Here's how the part is built. I have some questions about the finished solid (model axes, mm). Face numbers are marked on the shaded views. A direction names the side the tool comes from. Round coordinates to 2 decimals unless told otherwise and drop trailing zeros. Order: outer loops, then holes, each group sorted by start corner. A loop starts at its lowest first (then second) coordinate and runs counter-clockwise, first axis right, second up. Notation, with made-up numbers: M 57.25,-16 L 116.25,-16 A18 cw 116.25,-2 Z; hole C 88.5,49.25 d2. An arc over 180 degrees is marked long. Write each question's results on one line, items separated by ' | '. Start each with the question number.
```python
from build123d import *

# Parameters (mm, degrees)
EXTRUDE_THIN1_DEPTH            = 152.5
CONVERT_SOLID1_START           = -152.5
CONVERT_SOLID1_DEPTH           = 305
CONVERT_SOLID1_2_DEPTH         = 305
FILLET1_R                      = 2
F_6_5_6_5_DIAMETER_HOLE1_D     = 6.5
F_6_5_6_5_DIAMETER_HOLE2_D     = 6.5
F_6_5_6_5_DIAMETER_HOLE2_DEPTH = 497


# Read off the part's stored shape, not the designer's step: Convert-Solid1
with BuildPart() as part:
    # Sketch1 → Extrude-Thin1 (new, symmetric)
    with BuildSketch(Plane.XY):
        Polygon((-50, -60), (-50, 0), (50, 0), (50, -60), (46, -60), (46, -4), (-46, -4), (-46, -60), align=None)
    extrude(amount=EXTRUDE_THIN1_DEPTH, both=True)

    # Convert-Solid1 outline → Convert-Solid1 (cut)
    with BuildSketch(Plane.XY.offset(CONVERT_SOLID1_START)):
        with BuildLine():
            Line((50, 0), (44, 0))
            ThreePointArc((44, 0), (48.242640687, -1.757359313), (50, -6))
            Line((50, -6), (50, 0))
        make_face()
        with BuildLine():
            ThreePointArc((-50, -6), (-48.242640687, -1.757359313), (-44, 0))
            Line((-44, 0), (-50, 0))
            Line((-50, 0), (-50, -6))
        make_face()
    extrude(amount=CONVERT_SOLID1_DEPTH, mode=Mode.SUBTRACT)

    # Convert-Solid1 2 outline → Convert-Solid1 2 (add)
    with BuildSketch(Plane.XY.offset(CONVERT_SOLID1_START)):
        with BuildLine():
            Line((46, -4), (44, -4))
            ThreePointArc((44, -4), (45.414213562, -4.585786438), (46, -6))
            Line((46, -6), (46, -4))
        make_face()
        with BuildLine():
            ThreePointArc((-46, -6), (-45.414213562, -4.585786438), (-44, -4))
            Line((-44, -4), (-46, -4))
            Line((-46, -4), (-46, -6))
        make_face()
    extrude(amount=CONVERT_SOLID1_2_DEPTH)

    # Fillet1
    fillet1_edges = [part.edges().sort_by_distance(p)[0] for p in [
        (48, -60, 152.5),
        (48, -60, -152.5),
        (-48, -60, -152.5),
        (-48, -60, 152.5),
    ]]
    fillet(fillet1_edges, radius=FILLET1_R)

    # Ø6.5 (6.5) Diameter Hole1 (through all)
    with Locations(Plane(origin=(-244.5, 0, 0), x_dir=(0, 0, 1), z_dir=(0, 1, 0))):
        with Locations((-122.5, 244.5), (-62.5, 244.5), (62.5, 244.5), (122.5, 244.5)):
            Hole(F_6_5_6_5_DIAMETER_HOLE1_D / 2)

    # Ø6.5 (6.5) Diameter Hole2
    with Locations(Plane(origin=(-447, -38, 0), x_dir=(0, 0, 1), z_dir=(-1, 0, 0))):
        with Locations((-87.5, 8), (87.5, 8)):
            Hole(F_6_5_6_5_DIAMETER_HOLE2_D / 2, depth=F_6_5_6_5_DIAMETER_HOLE2_DEPTH)


solid = part.part
```
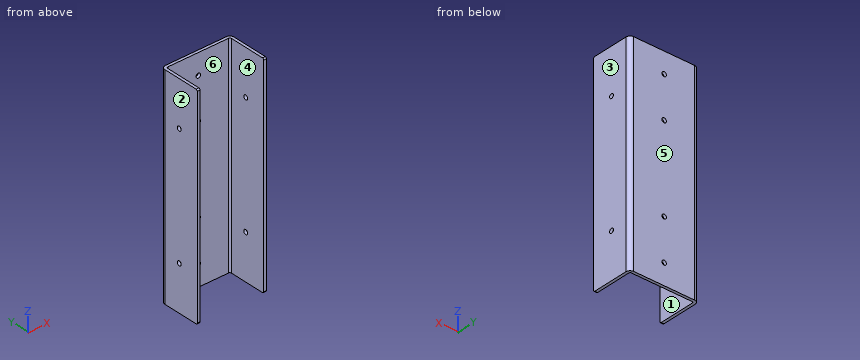
(1) Please list where these lines run through material, in increasing order: line 1 (X direction, y = -50, z = 97); line 2 (Y direction, x = -2.5, z = 126.5); line 3 (Y direction, x = -48, z = 87).
(2) I want a section at D-D on z = -87.5. Write out the boundary of the cut face in (x, y).
(3) I want a section at C-C on y = -19.5. Write out the boundary of the cut face in (x, z), and give its area (3 significant figures).
(4) I want a section at A-A on z = 62.5. Write out the boundary of the cut face in (x, y), and give its area (3 significant figures).
(5) On a 3-axis mill with a long thin cutter (end or side, diameter ignored), from which of +Z, -Z, +X, -X, +Y, -Y can I reach the whole of each face in a straight line? I mean the marked faces 1 and 2. Say none if no direction works.
(6) I want a section at B-B on x = 0. Write out the boundary of the cut face in (y, z).
(7) I'm going to push a flat-ended pin straight in: pin 1 Ø8.5 at (x, z) = (0, -62.5) entering from -Y. Where does the tip first touch, or does it pass through?
(8) If we mould it in two halves opening along X, with no side actions, what happens to the marked faces 3, 4, 5 and 6? For each: pulls with the +X half, pulls with the -X half, needs draft (parallel to the pull), parting line crosses it, or undercut.
Solutions:
1) line 1: -50 to -46, 46 to 50 | line 2: -4 to 0 | line 3: -60 to -33.21, -26.79 to -1.53
2) outline: M -50,-60 L -46,-60 L -46,-33.25 L -50,-33.25 Z; M -50,-26.75 L -46,-26.75 L -46,-6 A2 cw -44,-4 L 44,-4 A2 cw 46,-6 L 46,-26.75 L 50,-26.75 L 50,-6 A6 ccw 44,0 L -44,0 A6 ccw -50,-6 Z; M 46,-60 L 50,-60 L 50,-33.25 L 46,-33.25 Z
3) outline: M -50,-152.5 L -46,-152.5 L -46,152.5 L -50,152.5 Z; M 46,-152.5 L 50,-152.5 L 50,152.5 L 46,152.5 Z | area: 2,440 mm^2
4) outline: M -50,-60 L -46,-60 L -46,-6 A2 cw -44,-4 L -3.25,-4 L -3.25,0 L -44,0 A6 ccw -50,-6 Z; M 3.25,-4 L 44,-4 A2 cw 46,-6 L 46,-60 L 50,-60 L 50,-6 A6 ccw 44,0 L 3.25,0 Z | area: 808 mm^2
5) face 1: +Z, -Z, -Y | face 2: +Z, -Z, -X, +Y, -Y
6) outline: M -4,-152.5 L 0,-152.5 L 0,-125.75 L -4,-125.75 Z; M -4,-119.25 L 0,-119.25 L 0,-65.75 L -4,-65.75 Z; M -4,-59.25 L 0,-59.25 L 0,59.25 L -4,59.25 Z; M -4,65.75 L 0,65.75 L 0,119.25 L -4,119.25 Z; M -4,125.75 L 0,125.75 L 0,152.5 L -4,152.5 Z
7) pin 1: y = -4
8) face 3: pulls with the +X half | face 4: undercut | face 5: needs draft | face 6: undercut
